The figure shows three views and two pictorial views of one solid part (mm, origin at its lowest corner). Answer the questions. Give positions to 0.01 mm unless a question says otherwise; leave off trailing zeros. Order: outer loops, then holes, each group sorted by start corner. A loop starts at its lowest first (then second) coordinate and runs counter-clockwise, first axis right, second up. Notation, with made-up numbers: M 43.25,72.5 L 79.25,72.5 A6 ccw 79.25,76.5 Z; hole C 32.5,54 d9. An arc over 180 degrees is marked long. One line per item, written item: value.
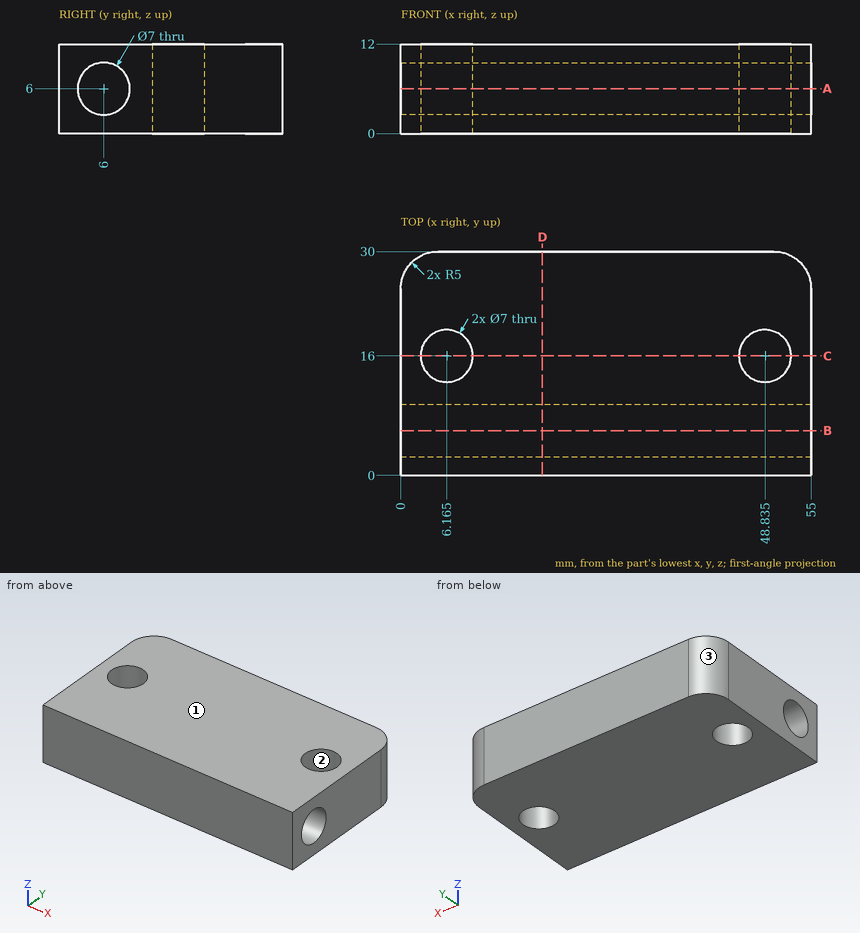
1) Find section B-B, the plane y = 6. Write down the section's boundary in (x, z).
Reported:
outline: M 0,0 L 55,0 L 55,2.5 L 0,2.5 Z; M 0,9.5 L 55,9.5 L 55,12 L 0,12 Z
2) Determine the mould class of the marked faces 1, 2 and 3 for opening direction Y: +Y half, -Y half, draft (parallel to the pull), parting line (faces both ways), or undercut.
Reported:
face 1: draft
face 2: undercut
face 3: +Y half
3) Find section D-D, the plane x = 19. Write down the section's boundary in (y, z).
Reported:
outline: M 0,0 L 30,0 L 30,12 L 0,12 Z; hole C 6,6 d7
4) Find section A-A, the plane z = 6. Write down the section's boundary in (x, y) (3 decimals).
Reported:
outline: M 0,0 L 55,0 L 55,2.5 L 0,2.5 Z; M 0,9.5 L 55,9.5 L 55,25 A5 ccw 50,30 L 5,30 A5 ccw 0,25 Z; hole C 6.165,16 d7; hole C 48.835,16 d7
5) Find section C-C, the plane y = 16. Write down the section's boundary in (x, z) (3 decimals), plus the area to 3 significant figures.
Reported:
outline: M 0,0 L 2.665,0 L 2.665,12 L 0,12 Z; M 9.665,0 L 45.335,0 L 45.335,12 L 9.665,12 Z; M 52.335,0 L 55,0 L 55,12 L 52.335,12 Z
area: 492 mm^2
6) Consider probe 1 along Y at (x, z) = (51, 4.25); probe 2 along Y at (x, z) = (52, 10.75); probe 3 along X at (y, z) = (13, 8). Determine where each line is inside the solid, lowest interval first.
Reported:
probe 1: y = 0 to 2.97, 9.03 to 13.25, 18.75 to 29.9
probe 2: y = 0 to 14.51, 17.49 to 29.58
probe 3: x = 0 to 4.36, 7.97 to 47.03, 50.64 to 55
